Check sheet for the drawn part. Datum: minimum x, y, z corner. Units: mm. Round coordinates to 2 decimals unless told otherwise and drop trailing zeros. Write each loop counter-clockwise with the first axis right and the second up, starting at its lowest first coordinate (ties: lowest second). Pieces come first, ordered by that corner, then holes. Notation, with made-up numbers: M 17,60.25 L 34,60.25 A14 ccw 34,80.25 Z; hole C 1.5,-2 d3. An arc over 180 degrees is marked long. One line per item, written item: value. Start each with the question number.
Item 1: Section check B-B, the plane x = 35. Record the cut outline in (y, z), then the cut area to 3 significant figures.
Item 2: Thickness scan on probe 1 along Y at (x, z) = (35, 2); probe 2 along Y at (x, z) = (48, 4.5); probe 3 along Y at (x, z) = (49.5, 3.25) (1 decimal). Record the ranges inside material, lowest first. Write a range as from..to.
Item 3: Draft check along X on the marked faces 1, 2 and 3. Enter one of: +X half, -X half, draft (parallel to the pull), parting line (faces both ways), or undercut.
Item 4: Gauge pin test, flat ends, axial feed: pin 1 (1.4 mm diameter, centred on x = 21, y = 57.5, fed in from +Z); pin 2 (3 mm diameter, centred on y = 47.5, z = 1, fed in from -X); pin 3 (1.5 mm diameter, centred on y = 61.5, z = 6, fed in from -X) (1 decimal). Record the tip position at first contact, or that the pin passes through.
Item 5: Section check D-D, the plane x = 48.5. Record the cut outline in (y, z), then the cut area to 3 significant figures.
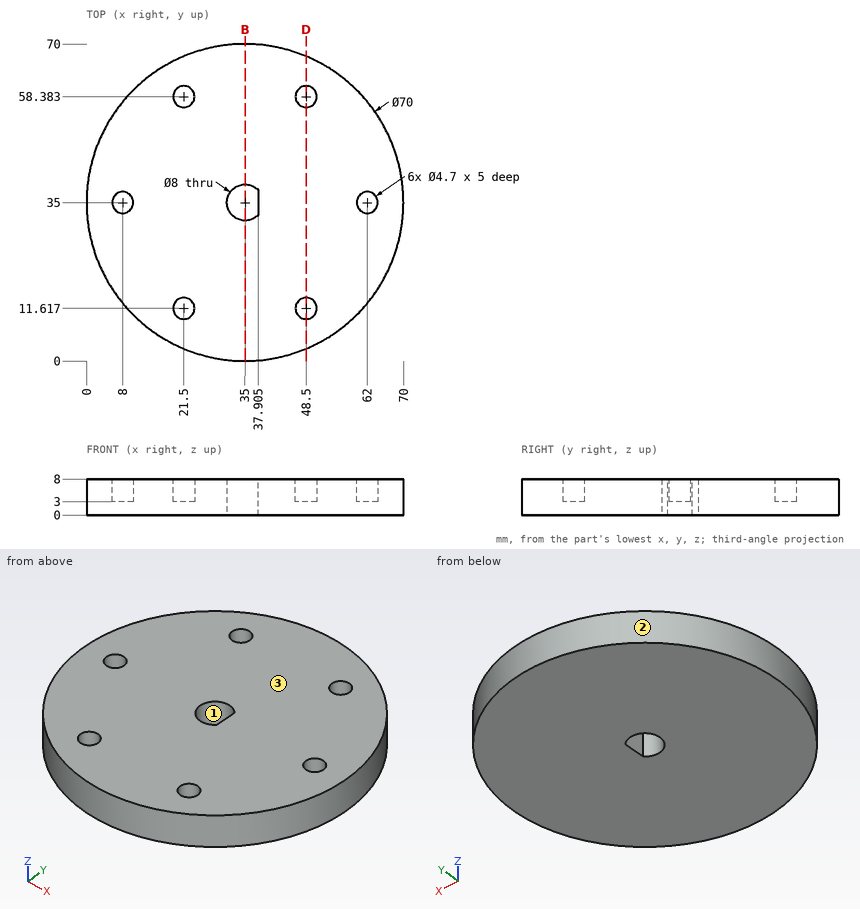
Response values:
1. outline: M 0,0 L 31,0 L 31,8 L 0,8 Z; M 39,0 L 70,0 L 70,8 L 39,8 Z
1. area: 496 mm2
2. probe 1: y = 0..31, 39..70
2. probe 2: y = 2.5..9.32, 13.91..56.09, 60.68..67.5
2. probe 3: y = 3.1..9.5, 13.7..56.3, 60.5..66.9
3. face 1: undercut
3. face 2: parting line
3. face 3: draft
4. pin 1: stops at z = 3
4. pin 2: stops at x = 1.77
4. pin 3: stops at x = 11.3
5. outline: M 2.71,0 L 67.29,0 L 67.29,8 L 60.73,8 L 60.73,3 L 56.03,3 L 56.03,8 L 13.97,8 L 13.97,3 L 9.27,3 L 9.27,8 L 2.71,8 Z
5. area: 470 mm2
